Could you check a few things on this model? Use its own coordinates, in mm. Face numbers are marked on the shaded views. Round coordinates to 2 decimals unless told otherwise and drop trailing zeros. Loops run counter-clockwise (first coordinate to the right, second up) from the corner with the lowest first, then second, coordinate; pieces in that order, holes last. Notation, with made-up numbers: (20.25, 53) - (56.25, 53) arc R32 cw to (56.25, 87) - close; hole circle Ø5 at (-21.5, 31). An arc over 180 degrees is marked (long way). Use one line per item in the form item = value.
```python
from build123d import *

# Parameters (mm, degrees)
SKETCH10_R                   = 3.175
BOSS_EXTRUDE1_DEPTH          = 12.7
SKETCH13_R                   = 3.175
TAPPED_HOLE_FOR_LID_DEPTH    = 12.7
CUT_TO_DECREASE_MASS_DEPTH   = 50.8
EIGTH_INCH_INTERNAL_FILLET_R = 3.175


with BuildPart() as part:
    # Sketch10 → Boss-Extrude1 (new body)
    with BuildSketch(Plane(origin=(0, 0, 0), x_dir=(1, 0, 0), z_dir=(0, 1, 0))):
        with BuildLine():
            Line((-7.543952838, -5.974068145), (-70.419757016, -68.718954232))
            Line((-70.419757016, -68.718954232), (-90.175514458, -48.954289951))
            ThreePointArc((-90.175514458, -48.954289951), (-93.011705319, -47.522259817), (-96.143902741, -48.0552028))
            ThreePointArc((-96.143902741, -48.0552028), (-110.274094487, -46.08424648), (-112.854196125, -32.052494517))
            ThreePointArc((-112.854196125, -32.052494517), (-100.207656711, -10.837422412), (-84.235041656, 8.001096953))
            ThreePointArc((-84.235041656, 8.001096953), (-65.363270894, 23.934411483), (-44.121885218, 36.536704058))
            ThreePointArc((-44.121885218, 36.536704058), (-30.095541538, 33.92736112), (-28.154041586, 19.79309193))
            ThreePointArc((-28.154041586, 19.79309193), (-28.693511967, 16.662012146), (-27.267396522, 13.822842611))
            Line((-27.267396522, 13.822842611), (-7.543952838, -5.974068145))
        make_face()
        with Locations(Location((-101.843613637, -37.280998562, 0), (0, 0, 270))):
            Circle(SKETCH10_R, mode=Mode.SUBTRACT)
        with Locations(Location((-38.9163423, 25.515247521, 0), (0, 0, 90))):
            Circle(SKETCH10_R, mode=Mode.SUBTRACT)
    extrude(amount=BOSS_EXTRUDE1_DEPTH)

    # Sketch13 → Tapped Hole for Lid (cut)
    with BuildSketch(Plane(origin=(-0.777086764, 0, -0.778708166), x_dir=(0.7078433221233256, 0, -0.7063694722490589), z_dir=(0.7063694722490589, 0, 0.7078433221233256))):
        with BuildLine():
            ThreePointArc((-88.862126184, 6.35), (-90.822106286, 9.283317516), (-94.282190214, 8.59506403))
            Line((-94.282190214, 8.59506403), (-89.792062153, 4.10493597))
            ThreePointArc((-89.792062153, 4.10493597), (-89.103808668, 5.134980102), (-88.862126184, 6.35))
        make_face()
        with BuildLine():
            Line((-89.792062153, 4.10493597), (-94.282190214, 8.59506403))
            ThreePointArc((-94.282190214, 8.59506403), (-94.282190214, 4.10493597), (-89.792062153, 4.10493597))
        make_face()
        with Locations(Location((-15.909836001, 6.35, 0), (0, 0, 180))):
            Circle(SKETCH13_R)
    extrude(amount=-TAPPED_HOLE_FOR_LID_DEPTH, mode=Mode.SUBTRACT)

    # Sketch14 → Cut to Decrease Mass (cut)
    with BuildSketch(Plane(origin=(-0.777086764, 0, -0.778708166), x_dir=(0.7078433221233256, 0, -0.7063694722490589), z_dir=(0.7063694722490589, 0, 0.7078433221233256))):
        with BuildLine():
            ThreePointArc((-79.337126184, 6.35), (-81.196998123, 1.859871939), (-85.687126184, 0))
            Line((-85.687126184, 0), (-22.259836001, 0))
            ThreePointArc((-22.259836001, 0), (-26.749964062, 1.859871939), (-28.609836001, 6.35))
            Line((-28.609836001, 6.35), (-79.337126184, 6.35))
        make_face()
    extrude(amount=-CUT_TO_DECREASE_MASS_DEPTH, mode=Mode.SUBTRACT)

    # Eigth Inch Internal Fillet
    # the kernel refuses this fillet: 3.175 mm, written as the material it adds along each edge
    with BuildSketch(Plane(origin=(-52.417132219, 6.35, -21.013480322), x_dir=(0.6718444169056685, -0.3148458040869803, -0.670445522858871), z_dir=(0.22286149992151785, 0.9491428341660821, -0.22239746447275088))) as eigth_inch_internal_fillet_piece_1_section:
        with BuildLine():
            CenterArc((6.35 + EIGTH_INCH_INTERNAL_FILLET_R, -EIGTH_INCH_INTERNAL_FILLET_R), EIGTH_INCH_INTERNAL_FILLET_R, 90, 90)
            Line((6.35 + EIGTH_INCH_INTERNAL_FILLET_R, 0), (6.35, 0))
            Line((6.35, 0), (6.35, -EIGTH_INCH_INTERNAL_FILLET_R))
        make_face()
    eigth_inch_internal_fillet_piece_1 = revolve(axis=Axis((-52.417132219, 6.35, -21.013480322), (-0.7063694722490589, 0, -0.7078433221233256)), revolution_arc=161.648494619, mode=Mode.PRIVATE)
    eigth_inch_internal_fillet_piece_1 = split(eigth_inch_internal_fillet_piece_1, bisect_by=Plane(origin=(-55.789501587, 0, -16.604615259), z_dir=(0, 1, 0)), keep=Keep.TOP, mode=Mode.PRIVATE)
    add(eigth_inch_internal_fillet_piece_1)
    with BuildSketch(Plane(origin=(-97.313716015, 6.35, 23.789621171), x_dir=(0.7078433221233247, 0, -0.7063694722490598), z_dir=(0, 1, 0))) as eigth_inch_internal_fillet_piece_2_section:
        with BuildLine():
            CenterArc((6.35 + EIGTH_INCH_INTERNAL_FILLET_R, -EIGTH_INCH_INTERNAL_FILLET_R), EIGTH_INCH_INTERNAL_FILLET_R, 90, 90)
            Line((6.35 + EIGTH_INCH_INTERNAL_FILLET_R, 0), (6.35, 0))
            Line((6.35, 0), (6.35, -EIGTH_INCH_INTERNAL_FILLET_R))
        make_face()
    eigth_inch_internal_fillet_piece_2 = revolve(axis=Axis((-97.313716015, 6.35, 23.789621171), (-0.7063694722490589, 0, -0.7078433221233256)), revolution_arc=161.648494619, mode=Mode.PRIVATE)
    eigth_inch_internal_fillet_piece_2 = split(eigth_inch_internal_fillet_piece_2, bisect_by=Plane(origin=(-92.897831362, 0, 20.426448518), z_dir=(0, 1, 0)), keep=Keep.TOP, mode=Mode.PRIVATE)
    add(eigth_inch_internal_fillet_piece_2)
    with BuildSketch(Plane(origin=(-51.293430945, 6.35, -22.134841859), x_dir=(0.7063694722490589, 0, 0.7078433221233255), z_dir=(-0.7078433221233256, 0, 0.7063694722490589))) as eigth_inch_internal_fillet_piece_3:
        with BuildLine():
            CenterArc((EIGTH_INCH_INTERNAL_FILLET_R, -EIGTH_INCH_INTERNAL_FILLET_R), EIGTH_INCH_INTERNAL_FILLET_R, 90, 90)
            Line((0, -EIGTH_INCH_INTERNAL_FILLET_R), (0, 0))
            Line((0, 0), (EIGTH_INCH_INTERNAL_FILLET_R, 0))
        make_face()
    extrude(amount=66.602290182)


solid = part.part
```
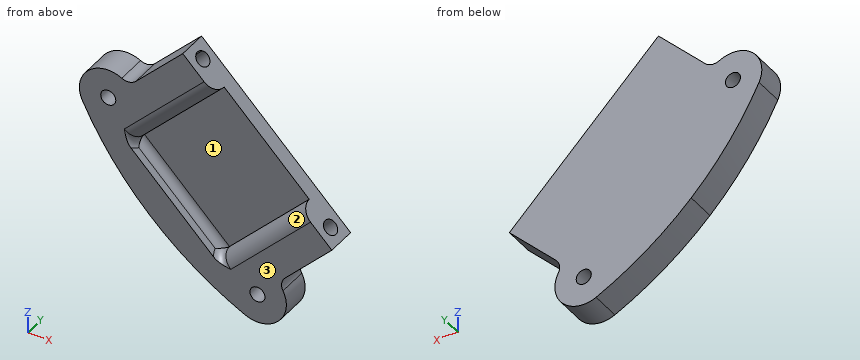
1. We'd pull the mould along Z, two halves only. Please class the marked faces 1, 2 and 3: +Z half, -Z half, draft (parallel to the pull), parting line (faces both ways), or undercut.
Solution:
face_1 = undercut
face_2 = +Z half
face_3 = draft
2. Please list where these lines run through material, in increasing order: line 1 along Y through (x, z) = (-66.5, 17.5); line 2 along Z through (x, y) = (-21.5, 4.25); line 3 along Z through (x, y) = (-38.5, 2.5).
Solution:
line_1 = 6.35 to 12.7
line_2 = -8.03 to 1.96, 4.35 to 18.45
line_3 = -37.7 to -28.66, -22.37 to 0.08
3. If we section it at A-A, the plane z = -24: Write out the boundary of the cut face in (x, y), plus the area to 3 significant figures.
Solution:
outline = (-65.27, 0) - (-41.71, 0) - (-41.71, 12.7) - (-65.27, 12.7) - close; (-36.13, 0) - (-26.82, 0) - (-26.82, 12.7) - (-36.13, 12.7) - close
area = 417 mm^2
4. If we section it at B-B, the plane y = 11: Count the separate pieces of the cut face and the enclosed holes in it, plus the area to 3 significant figures.
Solution:
separate_pieces = 1
enclosed_holes = 2
area = 5,910 mm^2
5. For P1, Ø3, axis at y = 4, z = 57.5, coming from the -X side; P2, Ø5.5, axis at x = -38.92, z = -25.52, coming from the -Y side; P3, Ø1, axis at x = -74.5, y = 11, coming from the -Z side; P4, Ø2, axis at y = 11, z = -25.5, coming from the -X side, each with a flat end and sliding along its axis, tell me the tip position at first contact or that it passes through.
Solution:
P1 = -83.13
P2 = through
P3 = -17.3
P4 = -64.56
